Design review of the part shown in the three views and the two pictorial views. Dimensions are in mm from the part's minimum x, y and z. Round coordinates to 2 decimals unless told otherwise and drop trailing zeros. Write each loop counter-clockwise with the first axis right and the second up, starting at its lowest first coordinate (ties: lowest second). Pieces come first, ordered by that corner, then holes. Notation, with made-up numbers: (29, -12) -> (80, -12) arc R16 ccw to (80, 16) -> close; hole circle Ø2 at (-20.75, 51.25). An arc over 180 degrees is marked (long way). Return JSON: item names as keys, results as strings. Group by question number.
1. Mouldability with a two-part tool opening along Z and no side actions: class the marked faces 1, 2, 3 and 4 as pulls with the +Z half, pulls with the -Z half, needs draft (parallel to the pull), parting line crosses it, or undercut.
2. For line 1 along Z through (x, y) = (6.75, 23); line 2 along X through (y, z) = (5.5, 84), list the stretches that pass through material, from the lowest coordinate up. Write a range as from..to.
3. Clearance check with flat-ended pins moving along their axes: P1, Ø1, axis at y = 8.5, z = 75.5, coming from the -X side; P2, Ø14, axis at x = 4, y = 19, coming from the -Z side. State where each tip first meets the part, or that it passes through.
4. Take a section at A-A, the plane x = 5.25. Write out the cut boundary in (y, z).
5. Take a section at C-C, the plane z = 76. Write out the cut boundary in (x, y).
6. Take a section at B-B, the plane y = 4.25. Write out the cut boundary in (x, z).
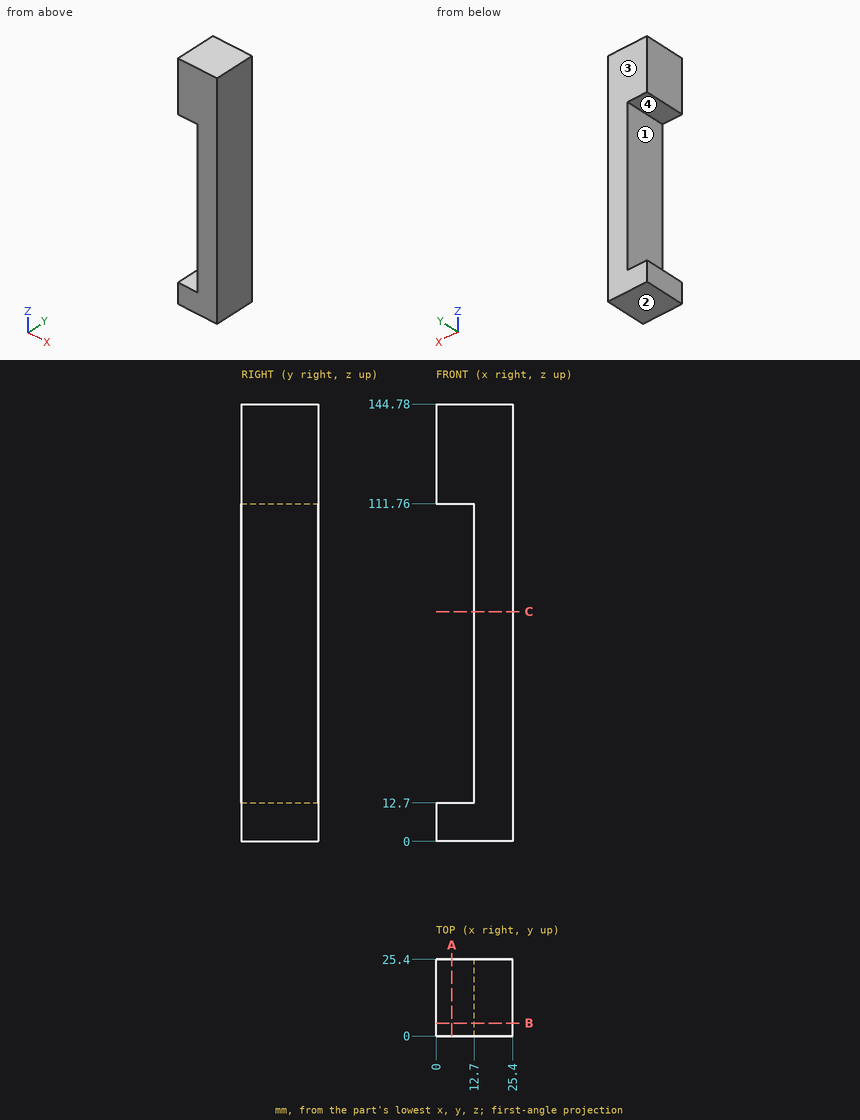
Output:
{
 "1": {"face 1": "undercut", "face 2": "pulls with the -Z half", "face 3": "needs draft", "face 4": "undercut"},
 "2": {"line 1": "z = 0..12.7, 111.76..144.78", "line 2": "x = 12.7..25.4"},
 "3": {"P1": "stops at x = 12.7", "P2": "stops at z = 0"},
 "4": {"outline": "(0, 0) -> (25.4, 0) -> (25.4, 12.7) -> (0, 12.7) -> close; (0, 111.76) -> (25.4, 111.76) -> (25.4, 144.78) -> (0, 144.78) -> close"},
 "5": {"outline": "(12.7, 0) -> (25.4, 0) -> (25.4, 25.4) -> (12.7, 25.4) -> close"},
 "6": {"outline": "(0, 0) -> (25.4, 0) -> (25.4, 144.78) -> (0, 144.78) -> (0, 111.76) -> (12.7, 111.76) -> (12.7, 12.7) -> (0, 12.7) -> close"}
}
